Read the model definition and answer for the solid it produces. Units are mm, in the model's axes. Face numbers are marked on the shaded views. A direction names the side the tool comes from. Coordinates: 2 decimals unless noted, no trailing zeros. Loops run counter-clockwise (first coordinate to the right, second up) from the corner with the lowest first, then second, coordinate; pieces in that order, holes last.
Q1. Section A-A (y = -525.5) is taken. Give the vertices of the cut face in (x, z).
Q2. Section B-B (x = -58.5) is taken. Give the vertices of the cut face in (y, z).
Q3. Section D-D (x = 135) is taken. Give the vertices of the cut face in (y, z).
Q4. Section C-C (z = -59.5) is taken. Give the vertices of the cut face in (x, y), then the cut area to 3 significant figures.
Q5. Which of the six approach directions +Z, -Z, +X, -X, +Y, -Y give full straight-line access (tool end or side, diameter ignored) to the marked faces 1, 2, 3 and 4?
Q6. A flat-ended cylindrical pin translates along its axis: P1, Ø5, axis at y = -367, z = -47.5, coming from the +X side. Find the tip coordinate at first contact, or state that the pin passes through.
Q7. The mould has two halves that part along Y. Classify the marked faces 5, 6 and 7: pulls with the +Y half, pulls with the -Y half, needs draft (parallel to the pull), parting line crosses it, or undercut.
Q8. Straight lines are drawn through the part: line 1 (Z direction, x = 83, y = -267.5); line 2 (X direction, y = -72, z = 13); line 3 (Y direction, x = 107.5, z = -47.5). For each, find the intervals that lie inside material, in ascending order.
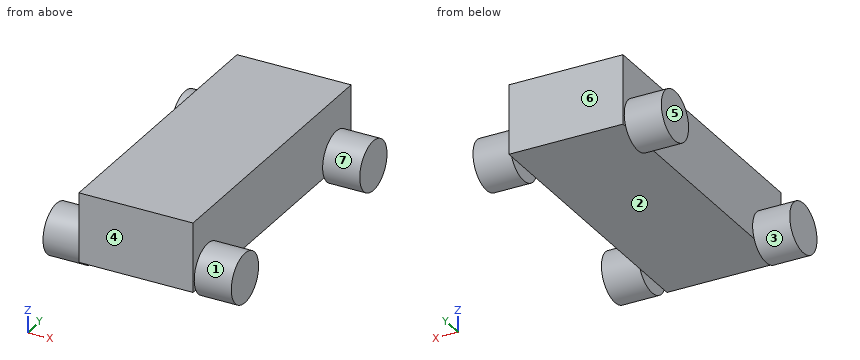
from build123d import *

# Parameters (mm, degrees)
F0_W     = 230.26
F0_H     = 140
F1_DEPTH = 580
F2_R     = 50
F3_DEPTH = 74.87
F4_R     = 50
F5_DEPTH = 74.87


with BuildPart() as f1:
    # F0 (on Front) → F1 (new body)
    with BuildSketch(Plane.XZ):
        with Locations((-11.937493, 2.456602)):
            Rectangle(F0_W, F0_H)
    extrude(amount=F1_DEPTH)

    # F2 (on face) → F3 (join)
    with BuildSketch(Plane(origin=(-127.067493, 0, 0), x_dir=(0, -1, 0), z_dir=(-1, 0, 0))):
        with Locations((54.5, -44.543398)):
            Circle(F2_R)
        with Locations((525.5, -44.543398)):
            Circle(F2_R)
    extrude(amount=F3_DEPTH)

    # F4 (on face) → F5 (join)
    with BuildSketch(Plane.YZ.offset(103.192507)):
        with Locations((-525.5, -44.543398)):
            Circle(F4_R)
        with Locations((-54.5, -44.543398)):
            Circle(F4_R)
    extrude(amount=F5_DEPTH)


solid = f1.part
Numbers:
1. outline: (-201.94, -94.54) - (-127.07, -94.54) - (-127.07, -67.54) - (103.19, -67.54) - (103.19, -94.54) - (178.06, -94.54) - (178.06, 5.46) - (103.19, 5.46) - (103.19, 72.46) - (-127.07, 72.46) - (-127.07, 5.46) - (-201.94, 5.46) - close
2. outline: (-580, -67.54) - (0, -67.54) - (0, 72.46) - (-580, 72.46) - close
3. outline: circle Ø100 at (-525.5, -44.54); circle Ø100 at (-54.5, -44.54)
4. outline: (-201.94, -573.21) - (-127.07, -573.21) - (-127.07, -580) - (103.19, -580) - (103.19, -573.21) - (178.06, -573.21) - (178.06, -477.79) - (103.19, -477.79) - (103.19, -102.21) - (178.06, -102.21) - (178.06, -6.79) - (103.19, -6.79) - (103.19, 0) - (-127.07, 0) - (-127.07, -6.79) - (-201.94, -6.79) - (-201.94, -102.21) - (-127.07, -102.21) - (-127.07, -477.79) - (-201.94, -477.79) - close
4. area: 162,000 mm2
5. face 1: +X
5. face 2: -Z, +Y, -Y
5. face 3: -X
5. face 4: +Z, -Z, +X, -X, -Y
6. P1: stops at x = 103.19
7. face 5: needs draft
7. face 6: pulls with the +Y half
7. face 7: undercut
8. line 1: z = -67.54 to 72.46
8. line 2: x = -127.07 to 103.19
8. line 3: y = -575.41 to -475.59, -104.41 to -4.59
